Could you check a few things on this model? Use its own coordinates, in mm. Round coordinates to 2 decimals unless told otherwise and drop trailing zeros. Order: outer loops, then holes, each group sorted by start corner. A loop starts at its lowest first (then second) coordinate and runs counter-clockwise, first axis right, second up. Notation, with made-up numbers: M 70.5,-12.75 L 92.5,-12.75 A5 cw 92.5,-6.75 Z; hole C 18,82 d9. An arc over 180 degrees is marked long. Write each question's results on one line, items separated by ' | '. Start each with the question number.
1. Suppose I cut it at A-A on y = -285.5. Write out the boundary of the cut face in (x, z).
2. Please list where these lines run through material, in increasing order: L1, parallel to Z at x = 0.75, y = -384; L2, parallel to X at y = -295, z = -0.5; L3, parallel to Z at x = 1, y = -169.5.
3. I'm going to push flat-ended pins straight in: pin 1 (1 mm diameter, centred on x = -3.5, y = -300, fed in from +Z); pin 2 (2 mm diameter, centred on y = -301, z = 3.5, fed in from -X); pin 3 (1 mm diameter, centred on y = -301.5, z = 6, fed in from +X); pin 4 (6 mm diameter, centred on y = -207.5, z = -3, fed in from -X). Where does each tip first touch, or does it pass through?
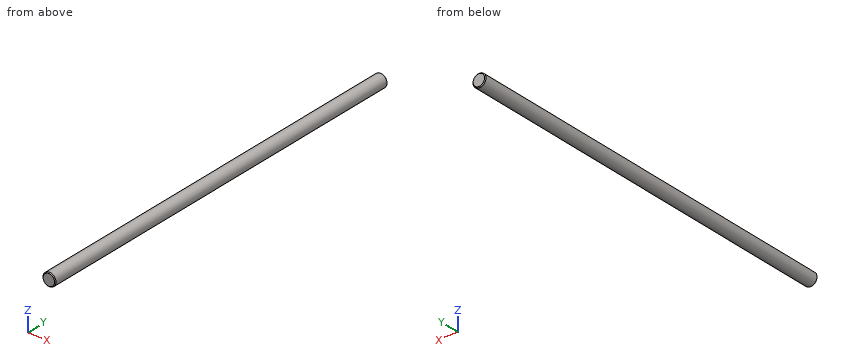
from build123d import *

# Parameters (mm, degrees)
SKETCH_R        = 8
PAD_DEPTH       = 500
CHAMFER_SIZE    = 1
CHAMFER001_SIZE = 1


with BuildPart() as part:
    # Sketch → Pad (new body)
    with BuildSketch(Plane.XZ):
        Circle(SKETCH_R)
    extrude(amount=PAD_DEPTH)

    # Chamfer
    chamfer_edges = [part.edges().sort_by_distance(p)[0] for p in [
        (-8, -500, 0),
    ]]
    chamfer(chamfer_edges, length=CHAMFER_SIZE)

    # Chamfer001
    chamfer001_edges = [part.edges().sort_by_distance(p)[0] for p in [
        (-8, 0, 0),
    ]]
    chamfer(chamfer001_edges, length=CHAMFER001_SIZE)


solid = part.part
Filled sheet:
1) outline: C 0,0 d16
2) L1: z = -7.96 to 7.96 | L2: x = -7.98 to 7.98 | L3: z = -7.94 to 7.94
3) pin 1: stops at z = 7.42 | pin 2: stops at x = -7.6 | pin 3: stops at x = 5.81 | pin 4: stops at x = -8
